from build123d import *

# Parameters (mm, degrees)
SKETCH1_W             = 82.45
SKETCH1_H             = 88
BOSS_EXTRUDE1_DEPTH   = 6
SKETCH2_W             = 82.45
SKETCH2_H             = 7
BOSS_EXTRUDE2_DEPTH   = 55
BOSS_EXTRUDE2_2_DEPTH = 55
SKETCH2_2_W           = 82.45
SKETCH2_2_H           = 7
BOSS_EXTRUDE3_DEPTH   = 6
SKETCH2_3_W           = 82.45
SKETCH2_3_H           = 7
BOSS_EXTRUDE4_DEPTH   = 6
BOSS_EXTRUDE5_DEPTH   = 7
BOSS_EXTRUDE7_DEPTH   = 7
SKETCH8_R             = 32.5
BOSS_EXTRUDE8_DEPTH   = 7
SKETCH9_R             = 35
BOSS_EXTRUDE9_DEPTH   = 2
SKETCH10_R            = 7.5
CUT_EXTRUDE3_DEPTH    = 7
SKETCH11_R            = 7.5
CUT_EXTRUDE4_DEPTH    = 7


with BuildPart() as part:
    # Sketch1 → Boss-Extrude1 (new body)
    with BuildSketch(Plane(origin=(0, 0, 0), x_dir=(1, 0, 0), z_dir=(0, 1, 0))):
        Rectangle(SKETCH1_W, SKETCH1_H)
    extrude(amount=-BOSS_EXTRUDE1_DEPTH)



with BuildPart() as body_2:
    # Sketch2 → Boss-Extrude2 (new body)
    with BuildSketch(Plane(origin=(0, 0, 0), x_dir=(1, 0, 0), z_dir=(0, 1, 0))):
        with Locations((0, 47.5)):
            Rectangle(SKETCH2_W, SKETCH2_H)
    extrude(amount=BOSS_EXTRUDE2_DEPTH)


with BuildPart() as body_3:
    # Sketch2 → Boss-Extrude2 2 (new body)
    with BuildSketch(Plane(origin=(0, 0, 0), x_dir=(1, 0, 0), z_dir=(0, 1, 0))):
        with Locations((0, -47.5)):
            Rectangle(SKETCH2_W, SKETCH2_H)
    extrude(amount=BOSS_EXTRUDE2_2_DEPTH)


with BuildPart() as part_1:
    add(part.part)

    add(body_2.part)  # Boss-Extrude3 merges body 2
    # Sketch2<2> → Boss-Extrude3 (add)
    with BuildSketch(Plane(origin=(0, 0, 0), x_dir=(1, 0, 0), z_dir=(0, 1, 0))):
        with Locations((0, 47.5)):
            Rectangle(SKETCH2_2_W, SKETCH2_2_H)
    extrude(amount=-BOSS_EXTRUDE3_DEPTH)


    add(body_3.part)  # Boss-Extrude4 merges body 3
    # Sketch2<3> → Boss-Extrude4 (add)
    with BuildSketch(Plane(origin=(0, 0, 0), x_dir=(1, 0, 0), z_dir=(0, 1, 0))):
        with Locations((0, -47.5)):
            Rectangle(SKETCH2_3_W, SKETCH2_3_H)
    extrude(amount=-BOSS_EXTRUDE4_DEPTH)

    # Sketch4 → Boss-Extrude5 (add)
    with BuildSketch(Plane.XY.offset(-44)):
        with BuildLine():
            Line((22.5, 55), (-22.5, 55))
            ThreePointArc((-22.5, 55), (0, 77.5), (22.5, 55))
        make_face()
    extrude(amount=-BOSS_EXTRUDE5_DEPTH)

    # Sketch5 → Boss-Extrude7 (add)
    with BuildSketch(Plane(origin=(0, 0, 44), x_dir=(-1, 0, 0), z_dir=(0, 0, -1))):
        with BuildLine():
            Line((22.5, 55), (-22.5, 55))
            ThreePointArc((-22.5, 55), (0, 77.5), (22.5, 55))
        make_face()
    extrude(amount=-BOSS_EXTRUDE7_DEPTH)

    # Sketch8 → Boss-Extrude8 (add)
    with BuildSketch(Plane.XZ.offset(6)):
        Circle(SKETCH8_R)
    extrude(amount=BOSS_EXTRUDE8_DEPTH)

    # Sketch9 → Boss-Extrude9 (add)
    with BuildSketch(Plane.XZ.offset(13)):
        Circle(SKETCH9_R)
    extrude(amount=BOSS_EXTRUDE9_DEPTH)

    # Sketch10 → Cut-Extrude3 (cut)
    with BuildSketch(Plane.XY.offset(-44)):
        with Locations((0, 55)):
            Circle(SKETCH10_R)
    extrude(amount=-CUT_EXTRUDE3_DEPTH, mode=Mode.SUBTRACT)

    # Sketch11 → Cut-Extrude4 (cut)
    with BuildSketch(Plane(origin=(0, 0, 44), x_dir=(-1, 0, 0), z_dir=(0, 0, -1))):
        with Locations((0, 55)):
            Circle(SKETCH11_R)
    extrude(amount=-CUT_EXTRUDE4_DEPTH, mode=Mode.SUBTRACT)


solid = part_1.part
Work out the finished part from the listing and answer in its coordinate system (mm). A direction names the side the tool comes from. Give positions to 0.01 mm unless a question says otherwise; leave off trailing zeros. Loops run counter-clockwise (first coordinate to the right, second up) from the corner with the lowest first, then second, coordinate; pieces in that order, holes last. Notation, with made-up numbers: (22, 0) -> (34, 0) arc R22 ccw to (34, 25) -> close; hole circle Ø6 at (-17, -22.5). An arc over 180 degrees is marked (long way). Use a Markdown table: item, result. Add a question column.
1) The part is cut by section A-A, the plane y = 44. Determine the outline of the cut face in (x, z) (3 decimals).
2) Which of the six approach directions +Z, -Z, +X, -X, +Y, -Y give full straight-line access (tool end or side, diameter ignored) to faces 1 (the cylindrical face through (-28, -14, -21)), 2 (the flat face through (-1, 0, -1)), 3 (the flat face through (32, 55, 47)), 4 (the cylindrical face through (31, -9.45, 9.76))?
3) The part is cut by section D-D, the plane y = 68. Determine the outline of the cut face in (x, z).
4) Consider line 1 along Z through (x, y) = (-5, 38.5); line 2 along Y through (x, z) = (0, -47.75); line 3 along Y through (x, z) = (1, -10.5). Determine where each line is inside the solid, lowest interval first.
5) The part is cut by section B-B, the plane x = 0. Determine the outline of the cut face in (y, z).
6) The part is cut by section C-C, the plane z = 0. Determine the outline of the cut face in (x, y) (3 decimals).
7) For a pull along Y with two mould halves and no side action, classify faces 5 (the flat face through (-1, 27, 51)), 6 (the cylindrical face through (1.63, 47.68, 47.45)), 7 (the flat face through (-32, 55, 47)) as +Y half, -Y half, draft (parallel to the pull), parting line (faces both ways), or undercut.
8) Each of these flat-tipped pins is pushed along its axis until it touches: P1, Ø5.5, axis at x = -30, z = -47.5, coming from the +Y side; P2, Ø2, axis at x = 3, z = 36.5, coming from the +Y side. Where does it stop, or does it pass through?
Reported:
| question | item | result |
|---|---|---|
| 1 | outline | (-41.225, -51) -> (41.225, -51) -> (41.225, -44) -> (-41.225, -44) -> close; (-41.225, 44) -> (41.225, 44) -> (41.225, 51) -> (-41.225, 51) -> close |
| 2 | face 1 | -Y |
| 2 | face 2 | +X, -X, +Y |
| 2 | face 3 | +Z, -Z, +X, +Y |
| 2 | face 4 | none |
| 3 | outline | (-18.36, -51) -> (18.36, -51) -> (18.36, -44) -> (-18.36, -44) -> close; (-18.36, 44) -> (18.36, 44) -> (18.36, 51) -> (-18.36, 51) -> close |
| 4 | line 1 | z = -51 to -44, 44 to 51 |
| 4 | line 2 | y = -6 to 47.5, 62.5 to 77.5 |
| 4 | line 3 | y = -15 to 0 |
| 5 | outline | (-15, -35) -> (-13, -35) -> (-13, -32.5) -> (-6, -32.5) -> (-6, -51) -> (47.5, -51) -> (47.5, -44) -> (0, -44) -> (0, 44) -> (47.5, 44) -> (47.5, 51) -> (-6, 51) -> (-6, 32.5) -> (-13, 32.5) -> (-13, 35) -> (-15, 35) -> close; (62.5, -51) -> (77.5, -51) -> (77.5, -44) -> (62.5, -44) -> close; (62.5, 44) -> (77.5, 44) -> (77.5, 51) -> (62.5, 51) -> close |
| 6 | outline | (-41.225, -6) -> (-32.5, -6) -> (-32.5, -13) -> (-35, -13) -> (-35, -15) -> (35, -15) -> (35, -13) -> (32.5, -13) -> (32.5, -6) -> (41.225, -6) -> (41.225, 0) -> (-41.225, 0) -> close |
| 7 | face 5 | draft |
| 7 | face 6 | undercut |
| 7 | face 7 | +Y half |
| 8 | P1 | stops at y = 55 |
| 8 | P2 | stops at y = 0 |
